Autodesk Inventor part; units mm, degrees
ref_plane "YZ Plane" through (0, 0, 0) normal (1, 0, 0) x (0, 1, 0)
ref_plane "XZ Plane" through (0, 0, 0) normal (0, 1, 0) x (-1, 0, 0)
ref_plane "XY Plane" through (0, 0, 0) normal (0, 0, 1) x (1, 0, 0)
sketch "Szkic1" plane through (0, 0, 0) normal (0, 1, 0) x (-1, 0, 0)
  line L0 (0, 0) -> (19.6, 0) construction
  line L1 (0, 0) -> (-19.6, 0) construction
  line L2 (0, 0) -> (0, 8.3) construction
  line L3 (0, 0) -> (0, -8.3) construction
  circle A0 centre (0, 0) radius 2.2 construction
  line L4 (0, -8.3) -> (0, -6.45) construction
  circle A1 centre (0, -6.45) radius 1.85 construction
  line L5 (0, 8.3) -> (0, 6.45) construction
  circle A2 centre (0, 6.45) radius 1.85 construction
  circle A3 centre (0, 0) radius 3.5 construction
  line L6 (19.6, 0) -> (17.45, 0) construction
  circle A4 centre (17.45, 0) radius 2.15 construction
  line L7 (-19.6, 0) -> (-17.45, 0) construction
  circle A5 centre (-17.45, 0) radius 2.15 construction
  line L8 (0, 3.5) -> (-17.6151, 2.1437) construction
  line L9 (0, -3.5) -> (-17.6151, -2.1437) construction
  line L10 (0, 3.5) -> (17.6151, 2.1437) construction
  line L11 (0, -3.5) -> (17.6151, -2.1437) construction
  arc A6 (1.85, 6.45) -> (-1.85, 6.45) centre (0, 6.45) ccw
  arc A7 (-1.85, -6.45) -> (1.85, -6.45) centre (0, -6.45) ccw
  arc A8 (17.6151, -2.1437) -> (17.6151, 2.1437) centre (17.45, 0) ccw
  arc A9 (-17.6151, 2.1437) -> (-17.6151, -2.1437) centre (-17.45, 0) ccw
  circle A10 centre (0, 0) radius 2.2
  line L12 (1.85, 6.45) -> (1.85, -6.45) construction
  line L13 (-1.85, 6.45) -> (-1.85, -6.45) construction
  line L14 (1.85, 3.3576) -> (1.85, 6.45)
  line L15 (-1.85, 3.3576) -> (-1.85, 6.45)
  line L16 (-1.85, -3.3576) -> (-1.85, -6.45)
  line L17 (1.85, -3.3576) -> (1.85, -6.45)
  line L18 (1.85, -3.3576) -> (17.6151, -2.1437)
  line L19 (1.85, 3.3576) -> (17.6151, 2.1437)
  line L20 (-1.85, 3.3576) -> (-17.6151, 2.1437)
  line L21 (-1.85, -3.3576) -> (-17.6151, -2.1437)
  dimension "d0" = 19.6
  dimension "d1" = 19.6
  dimension "d2" = 8.3
  dimension "d3" = 8.3
  dimension "d4" = 4.4
  dimension "d5" = 1.85
  dimension "d6" = 1.85
  dimension "d7" = 7
  dimension "d8" = 2.15
  dimension "d9" = 2.15
extrude "Wyciągnięcie proste1" add sketch "Szkic1" along normal blind 1.4
sketch "Szkic2" plane through (0, 0, 0) normal (0, -1, 0) x (1, 0, 0)
  circle A0 centre (0, 0) radius 2.2
  circle A1 centre (0, 0) radius 3.5
  dimension "d12" = 7
extrude "Wyciągnięcie proste2" add sketch "Szkic2" along normal blind 2.4
properties part number "orczyk_k"
Could you check a few things on this model? Use its own coordinates, in mm. A direction names the side the tool comes from. Give positions to 0.01 mm unless a question says otherwise; leave off trailing zeros. Order: outer loops, then holes, each group sorted by start corner. A loop starts at its lowest first (then second) coordinate and runs counter-clockwise, first axis right, second up. Notation, with made-up numbers: (-33.5, 55) -> (-6.5, 55) arc R24 cw to (-6.5, 67) -> close; hole circle Ø4 at (46, 6.5). An arc over 180 degrees is marked (long way). Answer in a Markdown table with one row per item. Add a question column.
Item 1: For faces 1 (the flat face through (1.85, 1, 5)), 2 (the flat face through (1.85, 1, -5)), 3 (the cylindrical face through (3.233, -1.183, 1.341)), 4 (the flat face through (-1.85, 1, -5)), 5 (the flat face through (-1.85, 1, 5)), which set-ups out of +Z, -Z, +X, -X, +Y, -Y let a thin tool reach every point of the face, with its end or its side?
Item 2: Imagine slicing it at D-D (z = 4.25). List the corners of the cut face in (x, y) for me, and give its area (3 significant figures).
Item 3: Imagine slicing it at A-A (z = 0). List the corners of the cut face in (x, y) for me, and give its area (3 significant figures).
Item 4: Imagine slicing it at C-C (y = 0.9). List the corners of the cut face in (x, z) for me, and give its area (3 significant figures).
Item 5: Please list where these lines run through material, in increasing order: probe 1 along Z at (x, y) = (0, 1.1); probe 2 along Z at (x, y) = (0, -0.7); probe 3 along Y at (x, z) = (-8, -0.5).
Item 6: Imagine slicing it at B-B (x = 0). List the corners of the cut face in (y, z) for me, and give its area (3 significant figures).
Item 7: I'm going to push flat-ended pins straight in: P1, Ø1.1, axis at y = 1, z = -5.5, coming from the +X side; P2, Ø1.5, axis at x = -5, z = -3.5, coming from the -Y side; P3, Ø0.7, axis at y = 0.5, z = -5, coming from the -X side. Where does each tip first touch, or does it pass through?
Result:
| question | item | result |
|---|---|---|
| 1 | face 1 | +Z, +X, +Y, -Y |
| 1 | face 2 | -Z, +X, +Y, -Y |
| 1 | face 3 | -Y |
| 1 | face 4 | -Z, -X, +Y, -Y |
| 1 | face 5 | +Z, -X, +Y, -Y |
| 2 | outline | (-1.85, 0) -> (1.85, 0) -> (1.85, 1.4) -> (-1.85, 1.4) -> close |
| 2 | area | 5.18 mm2 |
| 3 | outline | (-19.6, 0) -> (-3.5, 0) -> (-3.5, -2.4) -> (-2.2, -2.4) -> (-2.2, 1.4) -> (-19.6, 1.4) -> close; (2.2, -2.4) -> (3.5, -2.4) -> (3.5, 0) -> (19.6, 0) -> (19.6, 1.4) -> (2.2, 1.4) -> close |
| 3 | area | 55.0 mm2 |
| 4 | outline | (-17.62, -2.14) -> (-1.85, -3.36) -> (-1.85, -6.45) arc R1.85 ccw to (1.85, -6.45) -> (1.85, -3.36) -> (17.62, -2.14) arc R2.15 ccw to (17.62, 2.14) -> (1.85, 3.36) -> (1.85, 6.45) arc R1.85 ccw to (-1.85, 6.45) -> (-1.85, 3.36) -> (-17.62, 2.14) arc R2.15 ccw to start; hole circle Ø4.4 at (0, 0) |
| 4 | area | 230 mm2 |
| 5 | probe 1 | -8.3 to -2.2, 2.2 to 8.3 |
| 5 | probe 2 | -3.5 to -2.2, 2.2 to 3.5 |
| 5 | probe 3 | 0 to 1.4 |
| 6 | outline | (-2.4, -3.5) -> (0, -3.5) -> (0, -8.3) -> (1.4, -8.3) -> (1.4, -2.2) -> (-2.4, -2.2) -> close; (-2.4, 2.2) -> (1.4, 2.2) -> (1.4, 8.3) -> (0, 8.3) -> (0, 3.5) -> (-2.4, 3.5) -> close |
| 6 | area | 23.3 mm2 |
| 7 | P1 | x = 1.85 |
| 7 | P2 | y = 0 |
| 7 | P3 | x = -1.85 |
